from build123d import *

# Parameters (mm, degrees)
SKETCH_W     = 495
SKETCH_H     = 500
PAD_DEPTH    = 12
SKETCH001_W  = 372.304686
SKETCH001_H  = 400.790555
POCKET_DEPTH = 12.001


with BuildPart() as part:
    # Sketch → Pad (new body)
    with BuildSketch(Plane.YZ):
        with Locations((0, 250)):
            Rectangle(SKETCH_W, SKETCH_H)
    extrude(amount=PAD_DEPTH)

    # Sketch001 (on Face6 of Pad) → Pocket (cut, through all)
    with BuildSketch(Plane.YZ.offset(12)):
        Polygon((0, 495), (-10, 477.679492), (10, 477.679492), align=None)
        with Locations((0, 256.721156)):
            Rectangle(SKETCH001_W, SKETCH001_H)
    extrude(amount=-POCKET_DEPTH, mode=Mode.SUBTRACT)


solid = part.part
Work out the finished part from the listing and answer in its coordinate system (mm). A direction names the side the tool comes from. Coordinates: 2 decimals unless noted, no trailing zeros. Write each loop counter-clockwise with the first axis right and the second up, starting at its lowest first coordinate (ties: lowest second). Pieces come first, ordered by that corner, then holes. Notation, with made-up numbers: (-19.5, -25.75) - (9.5, -25.75) arc R13 ccw to (9.5, -17.75) - close; hole circle Ø9 at (-29.5, -19.75). An arc over 180 degrees is marked (long way). One line per question, with ' | ' between items.
1) Find section B-B, the plane x = 8.25. Determine the outline of the cut face in (y, z).
Checks:
outline: (-247.5, 0) - (247.5, 0) - (247.5, 500) - (-247.5, 500) - close; hole (-186.15, 56.33) - (186.15, 56.33) - (186.15, 457.12) - (-186.15, 457.12) - close; hole (-10, 477.68) - (10, 477.68) - (0, 495) - close
2) The mould has two halves that part along Z. Classify faces 3 (the face through (6, -247.5, 247)), 4 (the face through (6.08, -4.93, 486.46)), 5 (the face through (6, -3, 500)): +Z half, -Z half, draft (parallel to the pull), parting line (faces both ways), or undercut.
Checks:
face 3: draft | face 4: undercut | face 5: +Z half
3) Find section C-C, the plane y = -96.5. Determine the outline of the cut face in (x, z), and give its area (3 significant figures).
Checks:
outline: (0, 0) - (12, 0) - (12, 56.33) - (0, 56.33) - close; (0, 457.12) - (12, 457.12) - (12, 500) - (0, 500) - close | area: 1,190 mm2
4) Consider probe 1 along Z at (x, y) = (9.25, -25); probe 2 along Y at (x, z) = (0.75, 168). Determine where each line is inside the solid, lowest interval first. Write a range as [from, to].
Checks:
probe 1: [0, 56.33], [457.12, 500] | probe 2: [-247.5, -186.15], [186.15, 247.5]
5) Find section A-A, the plane z = 425.5. Determine the outline of the cut face in (x, y).
Checks:
outline: (0, -247.5) - (12, -247.5) - (12, -186.15) - (0, -186.15) - close; (0, 186.15) - (12, 186.15) - (12, 247.5) - (0, 247.5) - close
6) For faces 1 (the face through (0, -223, 254)), 2 (the face through (6, 186.152, 254)), determine the directions among +Z, -Z, +X, -X, +Y, -Y from which every point of the face is accessible in a straight line to the end or side of a thin tool.
Checks:
face 1: +Z, -Z, -X, +Y, -Y | face 2: +X, -X
